Source: CAD feature listing. Evaluate the final solid. Frame: model axes, mm. Coordinates: 2 decimals unless noted, no trailing zeros. Loops run counter-clockwise (first coordinate to the right, second up) from the corner with the lowest first, then second, coordinate; pieces in that order, holes last.
```python
from build123d import *

# Parameters (mm, degrees)
SKETCH1_R           = 20
BOSS_EXTRUDE1_DEPTH = 3
SKETCH3_R           = 2.735
CUT_EXTRUDE1_DEPTH  = 10
SKETCH4_R           = 0.5
CUT_EXTRUDE2_DEPTH  = 10


with BuildPart() as part:
    # Sketch1 → Boss-Extrude1 (new body)
    with BuildSketch(Plane.XY):
        Circle(SKETCH1_R)
    extrude(amount=BOSS_EXTRUDE1_DEPTH)

    # Sketch3 → Cut-Extrude1 (cut)
    with BuildSketch(Plane.XY.offset(3)):
        with Locations((0, -4.723654738)):
            Circle(SKETCH3_R)
        with Locations((9, 4.6)):
            Circle(SKETCH3_R)
        with Locations((-9, 4.6)):
            Circle(SKETCH3_R)
    extrude(amount=-CUT_EXTRUDE1_DEPTH, mode=Mode.SUBTRACT)

    # Sketch4 → Cut-Extrude2 (cut)
    with BuildSketch(Plane.XY.offset(3)):
        with Locations((0, 17)):
            Circle(SKETCH4_R)
    extrude(amount=-CUT_EXTRUDE2_DEPTH, mode=Mode.SUBTRACT)


solid = part.part
```
Q1. Section query D-D on z = 1.9. Return the cut outline in (x, y) (3 decimals), then the cut area to 3 significant figures.
Q2. Section query A-A on x = 0. Return the cut outline in (y, z), then the cut area to 3 significant figures.
Q3. Section query C-C on x = 9. Return the cut outline in (y, z) (3 decimals), then the cut area to 3 significant figures.
Q4. Draft query along Y for faces 1 (the flat face through (0, 0, 0)), 2 (the cylindrical face through (-6.474, 3.552, 1.521)), 3 (the cylindrical face through (-4.336, -19.524, 1.479)), 4 (the cylindrical face through (2.61, -3.9, 1.52)). Return one class per face: released by +Y, released by -Y, zero draft, split by the parting line, or undercut.
Q5. Material intervals for line 1 along Y through (x, z) = (0, 1.45); line 2 along Y through (x, z) = (-9.5, 2.45); line 3 along Y through (x, z) = (2.5, 1.35), sorted ascending.
Q6. First-contact query: pin 1 Ø1.5 at (x, z) = (-2, 2) entering from -Y; pin 2 Ø1.5 at (y, z) = (-11, 1) entering from +X. Flat tips, straight axial feed; report the tip coordinate or a pass-through.
Q7. Section query B-B on y = 4.6. Return the cut outline in (x, z) (3 decimals), then the cut area to 3 significant figures.
Resolved:
1. outline: circle Ø40 at (0, 0); hole circle Ø5.47 at (-9, 4.6); hole circle Ø5.47 at (0, -4.724); hole circle Ø1 at (0, 17); hole circle Ø5.47 at (9, 4.6)
1. area: 1,190 mm2
2. outline: (-20, 0) - (-7.46, 0) - (-7.46, 3) - (-20, 3) - close; (-1.99, 0) - (16.5, 0) - (16.5, 3) - (-1.99, 3) - close; (17.5, 0) - (20, 0) - (20, 3) - (17.5, 3) - close
2. area: 101 mm2
3. outline: (-17.861, 0) - (1.865, 0) - (1.865, 3) - (-17.861, 3) - close; (7.335, 0) - (17.861, 0) - (17.861, 3) - (7.335, 3) - close
3. area: 90.8 mm2
4. face 1: zero draft
4. face 2: undercut
4. face 3: split by the parting line
4. face 4: undercut
5. line 1: y = -20 to -7.46, -1.99 to 16.5, 17.5 to 20
5. line 2: y = -17.6 to 1.91, 7.29 to 17.6
5. line 3: y = -19.84 to -5.83, -3.61 to 19.84
6. pin 1: stops at y = -19.96
6. pin 2: stops at x = 17.17
7. outline: (-19.464, 0) - (-11.735, 0) - (-11.735, 3) - (-19.464, 3) - close; (-6.265, 0) - (6.265, 0) - (6.265, 3) - (-6.265, 3) - close; (11.735, 0) - (19.464, 0) - (19.464, 3) - (11.735, 3) - close
7. area: 84.0 mm2
